The model under review builds one solid part; all positions refer to its coordinate system, in mm. A direction names the side the tool comes from. Coordinates: 2 decimals unless noted, no trailing zeros. Order: outer loops, then holes, each group sorted by start corner. A loop starts at its lowest first (then second) coordinate and runs counter-clockwise, first axis right, second up. Notation, with made-up numbers: (-6, 37) -> (22, 37) arc R26 ccw to (22, 75) -> close; hole circle Ø8 at (-7, -36). An arc over 180 degrees is marked (long way). Use one line per item in the form item = value.
from build123d import *

# Parameters (mm, degrees)
BOSS_EXTRUDE1_DEPTH                                 = 2
SKETCH2_W                                           = 8
SKETCH2_H                                           = 73
BOSS_EXTRUDE2_DEPTH                                 = 4
CSK_FOR_M3_FLAT_COUNTERSUNK_HEAD_SCREW1_D           = 3.4
CSK_FOR_M3_FLAT_COUNTERSUNK_HEAD_SCREW1_DEPTH       = 10
CSK_FOR_M3_FLAT_COUNTERSUNK_HEAD_SCREW1_CSINK_D     = 6.3
CSK_FOR_M3_FLAT_COUNTERSUNK_HEAD_SCREW1_CSINK_ANGLE = 90
CSK_FOR_M3_FLAT_COUNTERSUNK_HEAD_SCREW1_TIP         = 1.021463052
SKETCH5_R                                           = 2.05
BOSS_EXTRUDE3_DEPTH                                 = 8
BOSS_EXTRUDE4_START                                 = -10
SKETCH6_R                                           = 2.05
BOSS_EXTRUDE4_DEPTH                                 = 10
BOSS_EXTRUDE5_START                                 = -5
SKETCH7_R                                           = 2.05
BOSS_EXTRUDE5_DEPTH                                 = 5
SKETCH13_R                                          = 2.1
CUT_EXTRUDE1_DEPTH                                  = 5
FILLET1_R                                           = 5
FILLET2_R                                           = 16
FILLET3_R                                           = 2
FILLET4_R                                           = 1
CHAMFER1_SIZE                                       = 0.5


# Read off the part's stored shape, not the designer's step: CSK for M3 Flat Countersunk Head Screw2
with BuildPart() as part:
    # Sketch1 → Boss-Extrude1 (new, symmetric)
    with BuildSketch(Plane.XY):
        with BuildLine():
            Line((-30, 14), (-16, 14))
            ThreePointArc((-16, 14), (0, 6), (16, 14))
            Line((16, 14), (30, 14))
            Line((30, 14), (30, -14))
            Line((30, -14), (-30, -14))
            Line((-30, -14), (-30, 14))
        make_face()
    extrude(amount=BOSS_EXTRUDE1_DEPTH, both=True)

    # Sketch2 → Boss-Extrude2 (add)
    with BuildSketch(Plane(origin=(0, 0, -2), x_dir=(-1, 0, 0), z_dir=(0, 0, -1))):
        with Locations((-20, 7.5)):
            Rectangle(SKETCH2_W, SKETCH2_H)
        with Locations((20, 7.5)):
            Rectangle(SKETCH2_W, SKETCH2_H)
    extrude(amount=-BOSS_EXTRUDE2_DEPTH)

    # CSK for M3 Flat Countersunk Head Screw1
    with Locations(Plane.XY.offset(2)):
        with Locations((25.5, -9.5), (-25.5, -9.5), (-12, 6), (12, 6)):
            CounterSinkHole(CSK_FOR_M3_FLAT_COUNTERSUNK_HEAD_SCREW1_D / 2, CSK_FOR_M3_FLAT_COUNTERSUNK_HEAD_SCREW1_CSINK_D / 2, depth=CSK_FOR_M3_FLAT_COUNTERSUNK_HEAD_SCREW1_DEPTH, counter_sink_angle=CSK_FOR_M3_FLAT_COUNTERSUNK_HEAD_SCREW1_CSINK_ANGLE)
            with Locations((0, 0, -(CSK_FOR_M3_FLAT_COUNTERSUNK_HEAD_SCREW1_DEPTH + CSK_FOR_M3_FLAT_COUNTERSUNK_HEAD_SCREW1_TIP / 2))):  # 118° drill point
                Cone(0, CSK_FOR_M3_FLAT_COUNTERSUNK_HEAD_SCREW1_D / 2, CSK_FOR_M3_FLAT_COUNTERSUNK_HEAD_SCREW1_TIP, mode=Mode.SUBTRACT)

    # Sketch5 → Boss-Extrude3 (add)
    # profile 1 of 2: a face of its own
    with BuildSketch(Plane(origin=(0, -29, 0), x_dir=(-1, 0, 0), z_dir=(0, -1, 0))):
        with BuildLine():
            Line((24, -2), (24, -9.561552813))
            ThreePointArc((24, -9.561552813), (20, -12), (16, -9.561552813))
            Line((16, -9.561552813), (16, -2))
            Line((16, -2), (24, -2))
        make_face()
        with Locations(Location((20, -7.5, 0), (0, 0, 90))):
            Circle(SKETCH5_R, mode=Mode.SUBTRACT)
    # profile 2 of 2: a face of its own
    with BuildSketch(Plane(origin=(0, -29, 0), x_dir=(-1, 0, 0), z_dir=(0, -1, 0))):
        with BuildLine():
            Line((-16, -9.561552813), (-16, -2))
            Line((-16, -2), (-24, -2))
            Line((-24, -2), (-24, -9.561552813))
            ThreePointArc((-24, -9.561552813), (-20, -12), (-16, -9.561552813))
        make_face()
        with Locations(Location((-20, -7.5, 0), (0, 0, 90))):
            Circle(SKETCH5_R, mode=Mode.SUBTRACT)
    extrude(amount=-BOSS_EXTRUDE3_DEPTH)

    # Sketch6 → Boss-Extrude4 (add)
    # profile 1 of 2: a face of its own
    with BuildSketch(Plane(origin=(0, 14, 0), x_dir=(1, 0, 0), z_dir=(0, 1, 0)).offset(BOSS_EXTRUDE4_START)):
        with BuildLine():
            Line((24, -2), (16, -2))
            Line((16, -2), (16, -9.561552813))
            ThreePointArc((16, -9.561552813), (20, -12), (24, -9.561552813))
            Line((24, -9.561552813), (24, -2))
        make_face()
        with Locations(Location((20, -7.5, 0), (0, 0, 90))):
            Circle(SKETCH6_R, mode=Mode.SUBTRACT)
    # profile 2 of 2: a face of its own
    with BuildSketch(Plane(origin=(0, 14, 0), x_dir=(1, 0, 0), z_dir=(0, 1, 0)).offset(BOSS_EXTRUDE4_START)):
        with BuildLine():
            Line((-24, -2), (-24, -9.561552813))
            ThreePointArc((-24, -9.561552813), (-20, -12), (-16, -9.561552813))
            Line((-16, -9.561552813), (-16, -2))
            Line((-16, -2), (-24, -2))
        make_face()
        with Locations(Location((-20, -7.5, 0), (0, 0, 90))):
            Circle(SKETCH6_R, mode=Mode.SUBTRACT)
    extrude(amount=BOSS_EXTRUDE4_DEPTH)

    # Sketch7 → Boss-Extrude5 (add)
    # profile 1 of 2: a face of its own
    with BuildSketch(Plane(origin=(0, 44, 0), x_dir=(1, 0, 0), z_dir=(0, 1, 0)).offset(BOSS_EXTRUDE5_START)):
        with BuildLine():
            Line((24, -2), (16, -2))
            Line((16, -2), (16, -9.561552813))
            ThreePointArc((16, -9.561552813), (20, -12), (24, -9.561552813))
            Line((24, -9.561552813), (24, -2))
        make_face()
        with Locations(Location((20, -7.5, 0), (0, 0, 90))):
            Circle(SKETCH7_R, mode=Mode.SUBTRACT)
    # profile 2 of 2: a face of its own
    with BuildSketch(Plane(origin=(0, 44, 0), x_dir=(1, 0, 0), z_dir=(0, 1, 0)).offset(BOSS_EXTRUDE5_START)):
        with BuildLine():
            Line((-24, -2), (-24, -9.561552813))
            ThreePointArc((-24, -9.561552813), (-20, -12), (-16, -9.561552813))
            Line((-16, -9.561552813), (-16, -2))
            Line((-16, -2), (-24, -2))
        make_face()
        with Locations(Location((-20, -7.5, 0), (0, 0, 90))):
            Circle(SKETCH7_R, mode=Mode.SUBTRACT)
    extrude(amount=BOSS_EXTRUDE5_DEPTH)

    # CSK for M3 Flat Countersunk Head Scr 2 → CSK for M3 Flat Countersunk Head Screw2 (revolve, cut)
    with BuildSketch(Plane(origin=(-20, 9, 0), x_dir=(1, 0, 0), z_dir=(0, -1, 0))):
        Polygon((1.7, 0.45), (1.7, 6.354821537), (0, 6.354821537), (0, -2), (4.15, -2), align=None)
    revolve(axis=Axis((-20, 9, 0), (0, 0, 1)), mode=Mode.SUBTRACT)

    # CSK for M3 Flat Countersunk Head Scr 3 o → CSK for M3 Flat Countersunk Head Scr 3 (revolve, cut)
    with BuildSketch(Plane(origin=(20, 9, 0), x_dir=(1, 0, 0), z_dir=(0, -1, 0))):
        Polygon((1.7, 0.45), (1.7, 6.354821537), (0, 6.354821537), (0, -2), (4.15, -2), align=None)
    revolve(axis=Axis((20, 9, 0), (0, 0, 1)), mode=Mode.SUBTRACT)

    # Sketch13 → Cut-Extrude1 (cut)
    with BuildSketch(Plane(origin=(0, 0, -2), x_dir=(-1, 0, 0), z_dir=(0, 0, -1))):
        with Locations((-20, 9)):
            Circle(SKETCH13_R)
        with Locations((20, 9)):
            Circle(SKETCH13_R)
    extrude(amount=-CUT_EXTRUDE1_DEPTH, mode=Mode.SUBTRACT)

    # Fillet1
    fillet1_edges = [part.edges().sort_by_distance(p)[0] for p in [
        (-30, 14, 0),
        (30, 14, 0),
        (30, -14, 0),
        (-30, -14, 0),
        (16, -14, 0),
        (-16, -14, 0),
    ]]
    fillet(fillet1_edges, radius=FILLET1_R)

    # Fillet2
    # the kernel refuses this fillet: 16 mm, written as the material it adds along each edge
    with BuildSketch(Plane(origin=(16, 14, 2), x_dir=(-0.894427190999915, -0.4472135954999595, 0), z_dir=(0, 0, -1))) as fillet2_piece_1:
        with BuildLine():
            CenterArc((10.733126292, 14.310835056), FILLET2_R, 206.565051177, 90)
            Line((-3.577708764, 7.155417528), (0, 0))
            ThreePointArc((0, 0), (8.94427191, -2.11145618), (17.88854382, 0))
        make_face()
    extrude(amount=4)
    with BuildSketch(Plane(origin=(-16, 14, 2), x_dir=(0.8944271909999153, -0.4472135954999591, 0), z_dir=(0, 0, -1))) as fillet2_piece_2:
        with BuildLine():
            CenterArc((10.733126292, -14.310835056), FILLET2_R, 63.434948823, 90)
            Line((-3.577708764, -7.155417528), (0, 0))
            ThreePointArc((0, 0), (8.94427191, 2.11145618), (17.88854382, 0))
        make_face()
    extrude(amount=4)

    # Fillet3
    fillet3_edges = [part.edges().sort_by_distance(p)[0] for p in [
        (-24, -25, 9.561552813),
        (-16, -25, 9.561552813),
        (16, -25, 9.561552813),
        (24, -25, 9.561552813),
        (16, 9, 9.561552813),
        (24, 9, 9.561552813),
        (-16, 9, 9.561552813),
        (-24, 9, 9.561552813),
        (16, 41.5, 9.561552813),
        (24, 41.5, 9.561552813),
        (-16, 41.5, 9.561552813),
        (-24, 41.5, 9.561552813),
    ]]
    fillet(fillet3_edges, radius=FILLET3_R)

    # Fillet4
    fillet4_edges = [part.edges().sort_by_distance(p)[0] for p in [
        (-24, 44, 3.5),
        (-20, 44, 12),
        (-16, 44, 3.5),
        (-16.102633404, 44, 9.632455532),
        (-23.897366596, 44, 9.632455532),
        (20, 44, 12),
        (16, 44, 3.5),
        (24, 44, 3.5),
        (16.102633404, 44, 9.632455532),
        (23.897366596, 44, 9.632455532),
        (-20, -29, 12),
        (-16, -29, 3.5),
        (-24, -29, 3.5),
        (-16.102633404, -29, 9.632455532),
        (-23.897366596, -29, 9.632455532),
        (20, -29, 12),
        (24, -29, 3.5),
        (16, -29, 3.5),
        (23.897366596, -29, 9.632455532),
        (16.102633404, -29, 9.632455532),
    ]]
    fillet(fillet4_edges, radius=FILLET4_R)

    # Chamfer1
    # the kernel refuses this chamfer: 0.5 mm, written as the material it adds along each edge
    with BuildSketch(Plane(origin=(16, 4, 2), x_dir=(-0.9996219169112968, 0, -0.02749587661058516), z_dir=(0, 1, 0)), Plane(origin=(-24, 4, 2), x_dir=(-0.9996219169112968, 0, -0.02749587661058968), z_dir=(0, 1, 0))) as chamfer1_piece_1:
        Polygon((CHAMFER1_SIZE * 0.999621916911, CHAMFER1_SIZE * 0.0274958766106), (-CHAMFER1_SIZE * 0.0274958766106, CHAMFER1_SIZE * 0.999621916911), (0, 0), align=None)
    extrude(amount=10)
    with BuildSketch(Plane(origin=(24, 4, 2), x_dir=(0.9996219169112968, 0, -0.027495876610585602), z_dir=(0, 1, 0)), Plane(origin=(-16, 4, 2), x_dir=(0.9996219169112968, 0, -0.027495876610590154), z_dir=(0, 1, 0))) as chamfer1_piece_2:
        Polygon((CHAMFER1_SIZE * 0.999621916911, -CHAMFER1_SIZE * 0.0274958766106), (-CHAMFER1_SIZE * 0.0274958766106, -CHAMFER1_SIZE * 0.999621916911), (0, 0), align=None)
    extrude(amount=10)


solid = part.part
Item 1: To check wall thickness, follow L1, parallel to Y at x = -20, z = 5; L2, parallel to X at y = -26.75, z = 7.5; L3, parallel to X at y = 9, z = 5.4. State the ranges of each line that lie inside material, in increasing order. Write a range as from..to.
Results found:
L1 = -29..-21, 4..7.3, 10.7..14, 39..44
L2 = -24..-22.05, -17.95..-16, 16..17.95, 22.05..24
L3 = -24..-21.7, -18.3..-16, 16..18.3, 21.7..24
Item 2: We need section B-B (x = 12). Write out the cut boundary in (y, z).
Results found:
outline = (-14.1, -2) -> (4.3, -2) -> (4.3, 0.55) -> (2.85, 2) -> (-14.1, 2) -> close; (7.7, -2) -> (11.42, -2) -> (11.42, 2) -> (9.15, 2) -> (7.7, 0.55) -> close
Item 3: Clearance check with flat-ended pins moving along their axes: pin 1 (4 mm diameter, centred on x = 20, y = 9, fed in from -Z); pin 2 (5.5 mm diameter, centred on y = 33, z = 3, fed in from -X); pin 3 (4 mm diameter, centred on x = 25.5, y = -9.5, fed in from +Z); pin 4 (5.5 mm diameter, centred on x = -25.5, y = -9.5, fed in from -Z). State where each tip first meets the part, or that it passes through.
Results found:
pin_1 = 3
pin_2 = -24
pin_3 = 0.85
pin_4 = -2
Item 4: We need section A-A (y = -15). Write out the cut boundary in (x, z).
Results found:
outline = (-24, -2) -> (-14, -2) -> (-14, 2) -> (-24, 2) -> close; (14, -2) -> (24, -2) -> (24, 2) -> (14, 2) -> close
Item 5: We need section C-C (z = 7.5). State how many separate pieces and enclosed holes the cut face has, plus the area to 3 significant figures.
Results found:
separate_pieces = 12
enclosed_holes = 0
area = 178 mm²
Item 6: Tool access review of faces 5 (the face through (-16, -25, 4)), 6 (the face through (-24, 32, 1)), 7 (the face through (20, 39, 5)): name each direction out of +Z, -Z, +X, -X, +Y, -Y from which nothing blocks a thin tool from reaching the whole face with its end or side.
Results found:
face_5 = +Z, -Z, -Y
face_6 = +Z, -Z, -X, +Y
face_7 = +Z, +X, -X
Item 7: Draft analysis for pull direction Y (two halves, no side actions). For faces 1 (the face through (20, 14, 5)), 2 (the face through (-14, -15, 0)), 3 (the face through (-20, 4, 5)), 4 (the face through (-20, 41, 12)), state which applies: released by +Y, released by -Y, zero draft, split by the parting line, or undercut.
Results found:
face_1 = undercut
face_2 = released by -Y
face_3 = undercut
face_4 = zero draft
